Can you work these out from the model? Positions are in its coordinate system, mm. A direction names the side the tool comes from. Give positions to 0.01 mm unless a question says otherwise; leave off trailing zeros. Loops run counter-clockwise (first coordinate to the right, second up) from the corner with the lowest first, then second, coordinate; pieces in that order, holes last. Notation, with made-up numbers: (25.25, -6.75) - (83.25, -6.75) arc R23 cw to (83.25, 30.25) - close; hole circle Ø10 at (27, -34.5). An arc over 180 degrees is marked (long way). Answer as a JSON object with one key per item and string values. Group by question number.
Item 1: Suppose I cut it at B-B on y = 68. Write out the boundary of the cut face in (x, z), and give its area (3 significant figures).
Item 2: Suppose I cut it at A-A on z = 2. Count the separate pieces of the cut face and the enclosed holes in it, and give its area (3 significant figures).
Item 3: Suppose I cut it at C-C on x = -18. Write out the boundary of the cut face in (y, z).
Item 4: Will these pins go through, and if not, where does the flat tip stop? pin 1 (7 mm diameter, centred on x = -25.98, y = 25, fed in from +Z); pin 2 (1.5 mm diameter, centred on x = -51.5, z = 2, fed in from +Y).
Item 5: Which directions (+Z, -Z, +X, -X, +Y, -Y) give clear straight access to the entire face, cutting with the end or side of a thin tool? Please do faces 1 (the flat face through (1, 84, 3)), 2 (the cylindrical face through (71, 95, 1)).
Item 6: Thinking about a two-plate mould opening in X: for faces 3 (the cylindrical face through (-22.165, 26.201, 1.479)), 4 (the flat face through (1, 84, 0)), 5 (the flat face through (-56.37, 49.32, 1.48)), which applies, pulls with the +X half, pulls with the -X half, needs draft (parallel to the pull), parting line crosses it, or undercut?
Item 7: Please list where these lines run through material, in increasing order: L1, parallel to Y at x = 0, z = 0.75; L2, parallel to Y at x = 26.5, z = 1.2; L3, parallel to X at y = 33, z = 0.55 (3 decimals).
Item 8: Suppose I cut it at D-D on y = 55. Write out the boundary of the cut face in (x, z), and give its area (3 significant figures).
from build123d import *

# Parameters (mm, degrees)
SKETCH1_R           = 20
SKETCH1_R_2         = 4
BOSS_EXTRUDE1_DEPTH = 3


with BuildPart() as part:
    # Sketch1 → Boss-Extrude1 (new body)
    with BuildSketch(Plane.XY):
        with BuildLine():
            Line((-32.287227439, 16.387822118), (-81.143613719, 83.193911059))
            ThreePointArc((-81.143613719, 83.193911059), (-82.591950965, 104.5143713), (-63.956450336, 114.972756547))
            Line((-63.956450336, 114.972756547), (63.956450336, 114.972756547))
            ThreePointArc((63.956450336, 114.972756547), (82.591950965, 104.5143713), (81.143613719, 83.193911059))
            Line((81.143613719, 83.193911059), (32.287227439, 16.387822118))
            ThreePointArc((32.287227439, 16.387822118), (0, 0), (-32.287227439, 16.387822118))
        make_face()
        with Locations((0, 40)):
            Circle(SKETCH1_R, mode=Mode.SUBTRACT)
        with Locations((0, 70)):
            Circle(SKETCH1_R_2, mode=Mode.SUBTRACT)
        with Locations((25.980762114, 55)):
            Circle(SKETCH1_R_2, mode=Mode.SUBTRACT)
        with Locations((25.980762114, 25)):
            Circle(SKETCH1_R_2, mode=Mode.SUBTRACT)
        with Locations((0, 10)):
            Circle(SKETCH1_R_2, mode=Mode.SUBTRACT)
        with Locations((-25.980762114, 25)):
            Circle(SKETCH1_R_2, mode=Mode.SUBTRACT)
        with Locations((-25.980762114, 55)):
            Circle(SKETCH1_R_2, mode=Mode.SUBTRACT)
        with BuildLine():
            Line((-65, 101), (-45, 101))
            ThreePointArc((-45, 101), (-39, 95), (-45, 89))
            Line((-45, 89), (-65, 89))
            ThreePointArc((-65, 89), (-71, 95), (-65, 101))
        make_face(mode=Mode.SUBTRACT)
        with BuildLine():
            Line((65, 101), (45, 101))
            ThreePointArc((45, 101), (39, 95), (45, 89))
            Line((45, 89), (65, 89))
            ThreePointArc((65, 89), (71, 95), (65, 101))
        make_face(mode=Mode.SUBTRACT)
    extrude(amount=BOSS_EXTRUDE1_DEPTH)


solid = part.part
Worked out:
{
 "1": {"outline": "(-70.03, 0) - (-3.46, 0) - (-3.46, 3) - (-70.03, 3) - close; (3.46, 0) - (70.03, 0) - (70.03, 3) - (3.46, 3) - close", "area": "399 mm2"},
 "2": {"separate pieces": "1", "enclosed holes": "9", "area": "11,300 mm2"},
 "3": {"outline": "(4.28, 0) - (31.28, 0) - (31.28, 3) - (4.28, 3) - close; (48.72, 0) - (114.97, 0) - (114.97, 3) - (48.72, 3) - close"},
 "4": {"pin 1": "passes through", "pin 2": "stops at y = 114.97"},
 "5": {"face 1": "+Z, +X, -X, +Y, -Y", "face 2": "+Z, -Z"},
 "6": {"face 3": "undercut", "face 4": "needs draft", "face 5": "pulls with the -X half"},
 "7": {"L1": "y = 0 to 6, 14 to 20, 60 to 66, 74 to 114.97", "L2": "y = 10.04 to 21.03, 28.97 to 51.03, 58.97 to 114.97", "L3": "x = -44.436 to -18.735, 18.735 to 44.436"},
 "8": {"outline": "(-60.52, 0) - (-29.98, 0) - (-29.98, 3) - (-60.52, 3) - close; (-21.98, 0) - (-13.23, 0) - (-13.23, 3) - (-21.98, 3) - close; (13.23, 0) - (21.98, 0) - (21.98, 3) - (13.23, 3) - close; (29.98, 0) - (60.52, 0) - (60.52, 3) - (29.98, 3) - close", "area": "236 mm2"}
}
